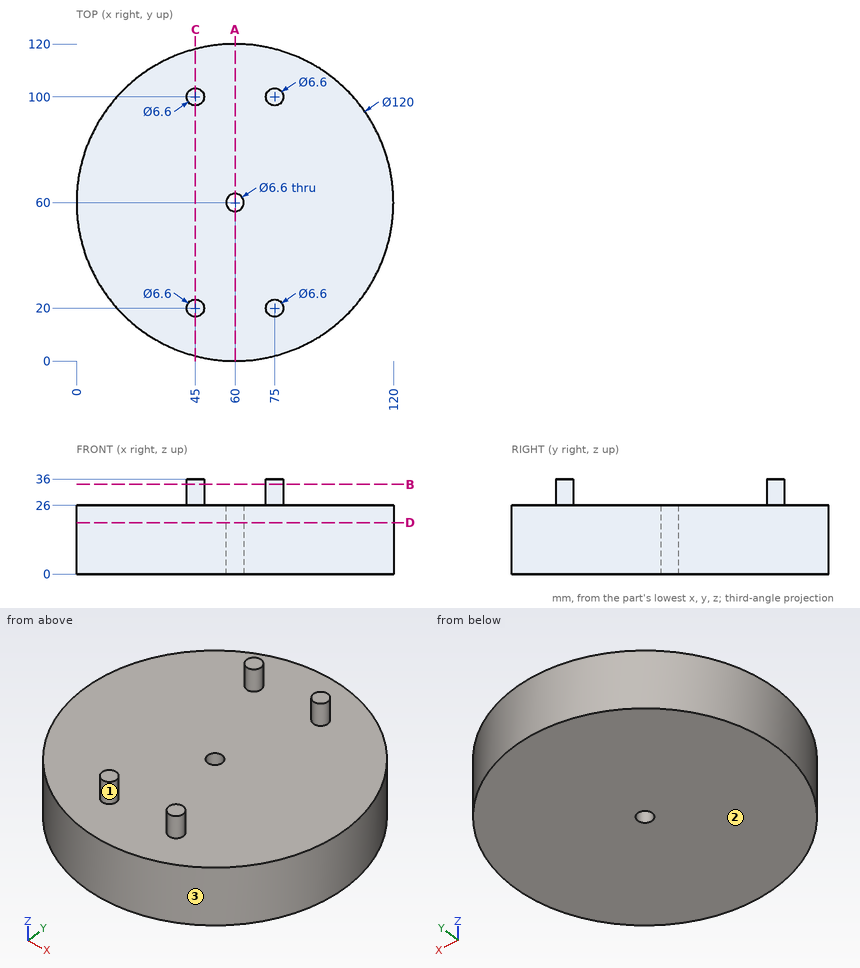
Here's the drawing with two shaded views (mm, measured from the low corner). I have some questions. Round coordinates to 2 decimals unless told otherwise and drop trailing zeros. Write each loop counter-clockwise with the first axis right and the second up, starting at its lowest first coordinate (ties: lowest second). Pieces come first, ordered by that corner, then holes. Notation, with made-up numbers: M -7,39.25 L 28,39.25 A12 cw 28,43.25 Z; hole C -14,39 d1. An arc over 180 degrees is marked long. Answer in a Markdown table with one row per item. Add a question column.
Q1. Imagine slicing it at B-B (z = 34). Please give me the cut outline in (x, y), then the cut area to 3 significant figures.
Q2. If we mould it in two halves opening along X, with no side actions, what happens to the marked faces 1, 2 and 3? For each: +X half, -X half, draft (parallel to the pull), parting line (faces both ways), or undercut.
Q3. If I drill on line 1 (Y direction, x = 60, z = 18); line 2 (Z direction, x = 80.5, y = 86.5); line 3 (Y direction, x = 80, z = 22), over which ranges is the centre line in solid material (lowest first)? Write a range as from..to.
Q4. Imagine slicing it at C-C (x = 45). Please give me the cut outline in (y, z), then the cut area to 3 significant figures.
Q5. Imagine slicing it at A-A (x = 60). Please give me the cut outline in (y, z).
Q6. Imagine slicing it at D-D (z = 19.5). Please give me the cut outline in (x, y), then the cut area to 3 significant figures.
Q7. Will these pins go through, and if not, where does the flat tip stop? pin 1 Ø5 at (y, z) = (85, 3.5) entering from +X; pin 2 Ø12 at (x, z) = (72, 17.5) entering from +Y; pin 3 Ø4 at (x, z) = (83, 21.5) entering from +Y (3 decimals).
Values:
| question | item | result |
|---|---|---|
| 1 | outline | C 45,20 d6.6; C 45,100 d6.6; C 75,20 d6.6; C 75,100 d6.6 |
| 1 | area | 137 mm^2 |
| 2 | face 1 | undercut |
| 2 | face 2 | draft |
| 2 | face 3 | parting line |
| 3 | line 1 | 0..56.7, 63.3..120 |
| 3 | line 2 | 0..26 |
| 3 | line 3 | 3.43..116.57 |
| 4 | outline | M 1.91,0 L 118.09,0 L 118.09,26 L 103.3,26 L 103.3,36 L 96.7,36 L 96.7,26 L 23.3,26 L 23.3,36 L 16.7,36 L 16.7,26 L 1.91,26 Z |
| 4 | area | 3,150 mm^2 |
| 5 | outline | M 0,0 L 56.7,0 L 56.7,26 L 0,26 Z; M 63.3,0 L 120,0 L 120,26 L 63.3,26 Z |
| 6 | outline | C 60,60 d120; hole C 60,60 d6.6 |
| 6 | area | 11,300 mm^2 |
| 7 | pin 1 | x = 115.62 |
| 7 | pin 2 | y = 119.7 |
| 7 | pin 3 | y = 116.205 |
